from build123d import *

# Parameters (mm, degrees)
F0_R           = 5
F0_R_2         = 6
F0_R_3         = 28.5
F1_DEPTH       = 30
F2_SIZE        = 4
F4_D           = 12
F4_DEPTH       = 35
F4_CSINK_D     = 13
F4_CSINK_ANGLE = 90
F4_TIP         = 3.6051637142


with BuildPart() as f1:
    # F0 (on Front) → F1 (new body)
    with BuildSketch(Plane.XZ):
        with BuildLine():
            Line((65, -380), (65, 0))
            ThreePointArc((65, 0), (45.9619407771, 45.9619407771), (0, 65))
            ThreePointArc((0, 65), (-45.9619407771, 45.9619407771), (-65, 0))
            Line((-65, 0), (-65, -380))
            ThreePointArc((-65, -380), (-70.8578643763, -394.1421356237), (-85, -400))
            Line((-85, -400), (-130, -400))
            ThreePointArc((-130, -400), (-144.1421356237, -405.8578643763), (-150, -420))
            Line((-150, -420), (-150, -463))
            Line((-150, -463), (-115, -463))
            Line((-115, -463), (-115, -490))
            Line((-115, -490), (115, -490))
            Line((115, -490), (115, -463))
            Line((115, -463), (150, -463))
            Line((150, -463), (150, -420))
            ThreePointArc((150, -420), (144.1421356237, -405.8578643763), (130, -400))
            Line((130, -400), (85, -400))
            ThreePointArc((85, -400), (70.8578643763, -394.1421356237), (65, -380))
        make_face()
        with Locations((-35.9210244843, -35.9210244843)):
            Circle(F0_R, mode=Mode.SUBTRACT)
        with Locations((-50, 0)):
            Circle(F0_R_2, mode=Mode.SUBTRACT)
        with Locations((-35.9210244843, 35.9210244843)):
            Circle(F0_R, mode=Mode.SUBTRACT)
        with Locations((0, -50)):
            Circle(F0_R_2, mode=Mode.SUBTRACT)
        with Locations((35.9210244843, -35.9210244843)):
            Circle(F0_R, mode=Mode.SUBTRACT)
        Circle(F0_R_3, mode=Mode.SUBTRACT)
        with Locations((0, 50)):
            Circle(F0_R_2, mode=Mode.SUBTRACT)
        with Locations((35.9210244843, 35.9210244843)):
            Circle(F0_R, mode=Mode.SUBTRACT)
        with Locations((50, 0)):
            Circle(F0_R_2, mode=Mode.SUBTRACT)
    extrude(amount=F1_DEPTH)

    # F2
    f2_edges = [f1.edges().sort_by_distance(p)[0] for p in [
        (-40.921024, -30, 35.921024),
        (-6, -30, 50),
        (30.921024, -30, 35.921024),
        (44, -30, 0),
        (30.921024, -30, -35.921024),
        (-6, -30, -50),
        (-40.921024, -30, -35.921024),
        (-56, -30, 0),
    ]]
    chamfer(f2_edges, length=F2_SIZE)

    # F4
    with Locations(Plane(origin=(0, 0, -463), x_dir=(1, 0, 0), z_dir=(0, 0, -1))):
        with Locations((-140, 15), (140, 15)):
            CounterSinkHole(F4_D / 2, F4_CSINK_D / 2, depth=F4_DEPTH, counter_sink_angle=F4_CSINK_ANGLE)
            with Locations((0, 0, -(F4_DEPTH + F4_TIP / 2))):  # 118° drill point
                Cone(0, F4_D / 2, F4_TIP, mode=Mode.SUBTRACT)


solid = f1.part
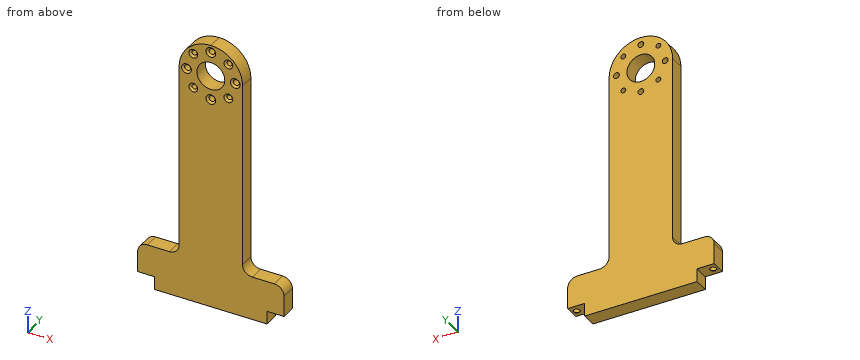
Read the model definition and answer for the solid it produces. Units are mm, in the model's axes. Coordinates: 2 decimals unless noted, no trailing zeros. Loops run counter-clockwise (first coordinate to the right, second up) from the corner with the lowest first, then second, coordinate; pieces in that order, holes last. Notation, with made-up numbers: (-32, 37) -> (6, 37) arc R31 cw to (6, 62) -> close; hole circle Ø7 at (-32.5, 65.5). An arc over 180 degrees is marked (long way). Answer in a Markdown table with one row per item.
Item 1: A cutting plane is placed at A-A on z = -50. Determine the outline of the cut face in (x, y), plus the area to 3 significant figures.
Returned:
| item | result |
|---|---|
| outline | (-65, -30) -> (-10, -30) -> (-6, -26) -> (-6, 0) -> (-65, 0) -> close; (6, -26) -> (10, -30) -> (65, -30) -> (65, 0) -> (6, 0) -> close |
| area | 3,520 mm^2 |
Item 2: Straight lines are drawn through the part: line 1 along Z through (x, y) = (-39, -24.5); line 2 along X through (y, z) = (-13, -440.5); line 3 along Z through (x, y) = (21, -2.5). For each, find the intervals that lie inside material, in ascending order. Write a range as [from, to].
Returned:
| item | result |
|---|---|
| line 1 | z = [-490, -39.86], [-31.98, 31.98], [39.86, 52] |
| line 2 | x = [-150, -145.66], [-134.34, 134.34], [145.66, 150] |
| line 3 | z = [-490, -19.27], [19.27, 61.51] |
Item 3: A cutting plane is placed at C-C on z = -241.5. Determine the outline of the cut face in (x, y).
Returned:
| item | result |
|---|---|
| outline | (-65, -30) -> (65, -30) -> (65, 0) -> (-65, 0) -> close |
Item 4: A cutting plane is placed at B-B on x = 50. Determine the outline of the cut face in (y, z).
Returned:
| item | result |
|---|---|
| outline | (-30, -490) -> (0, -490) -> (0, -6) -> (-26, -6) -> (-30, -10) -> close; (-30, 10) -> (-26, 6) -> (0, 6) -> (0, 41.53) -> (-30, 41.53) -> close |
Item 5: Each of these flat-tipped pins is pushed along its axis until it touches: P1, Ø1.5, axis at y = -25.5, z = -159.5, coming from the +X side; P2, Ø15.5, axis at x = 0, z = -50, coming from the -Y side; P3, Ø9, axis at x = -137.5, y = -14.5, coming from the -Z side; P4, Ø8, axis at x = -35.92, z = -35.92, coming from the +Y side. Where does it stop, or does it pass through?
Returned:
| item | result |
|---|---|
| P1 | stops at x = 65 |
| P2 | stops at y = -27.75 |
| P3 | stops at z = -463 |
| P4 | passes through |
